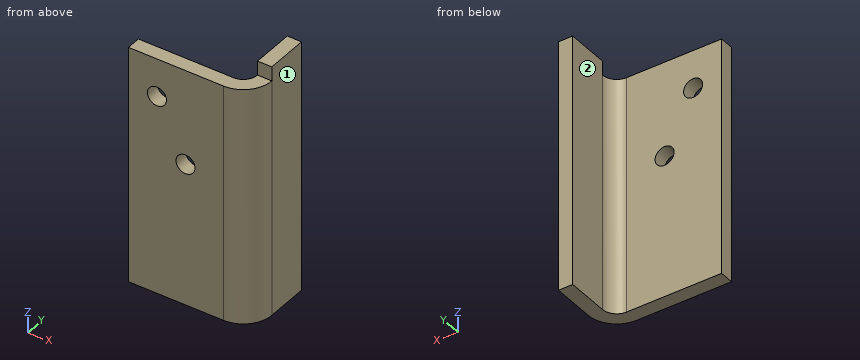
from build123d import *

# Parameters (mm, degrees)
SKETCH1_W               = 20
SKETCH1_H               = 50
SKETCH1_R               = 2
BASE_FLANGE1_DEPTH      = 3
EDGE_FLANGE1_DEPTH      = 50
EDGE_FLANGE1_START      = 3
EDGE_FLANGE1_PROFILE_W  = 53
EDGE_FLANGE1_PROFILE_H  = 9
EDGE_FLANGE1_FLAT_DEPTH = 3


# Sheet-metal steps are written as plain solids
with BuildPart() as part:
    # Sketch1 → Base-Flange1 (new body)
    with BuildSketch(Plane(origin=(0, 0, 0), x_dir=(1, 0, 0), z_dir=(0, 1, 0))):
        Rectangle(SKETCH1_W, SKETCH1_H)
        with Locations(Location((-4, 17, 0), (0, 0, 270))):
            Circle(SKETCH1_R, mode=Mode.SUBTRACT)
        with Locations(Location((2, 5, 0), (0, 0, 270))):
            Circle(SKETCH1_R, mode=Mode.SUBTRACT)
    extrude(amount=-BASE_FLANGE1_DEPTH)

    # Edge-Flange1 bend section (across the edge) → Edge-Flange1 (add)
    with BuildSketch(Plane(origin=(13, 0, 25), x_dir=(-1, 0, 0), z_dir=(0, 0, -1))):
        with BuildLine():
            Line((-3, 3), (0, 3))
            ThreePointArc((0, 3), (0.878679656, 0.878679656), (3, 0))
            Line((3, 0), (3, -3))
            ThreePointArc((3, -3), (-1.242640687, -1.242640687), (-3, 3))
        make_face()
    extrude(amount=EDGE_FLANGE1_DEPTH)

    # Edge-Flange1 profile (on flange) → Edge-Flange1 flat (add)
    with BuildSketch(Plane(origin=(13, 0, 0), x_dir=(0, 0, -1), z_dir=(1, 0, 0)).offset(EDGE_FLANGE1_START)):
        with Locations((1.5, 7.5)):
            Rectangle(EDGE_FLANGE1_PROFILE_W, EDGE_FLANGE1_PROFILE_H)
    extrude(amount=-EDGE_FLANGE1_FLAT_DEPTH)


with BuildPart() as body_2:
    # Mirror1: mirrored copy
    add(part.part.mirror(Plane(origin=(14.5, 7.5, -28), x_dir=(1, 0, 0), z_dir=(0, 0, -1))))


solid = body_2.part
The model under review builds one solid part; all positions refer to its coordinate system, in mm. Face numbers are marked on the shaded views. A direction names the side the tool comes from. Round coordinates to 2 decimals unless told otherwise and drop trailing zeros. Write each loop counter-clockwise with the first axis right and the second up, starting at its lowest first coordinate (ties: lowest second). Pieces come first, ordered by that corner, then holes. Notation, with made-up numbers: (40.5, 22.25) -> (89.5, 22.25) arc R29 ccw to (89.5, 52.25) -> close; hole circle Ø10 at (62, -10). An arc over 180 degrees is marked (long way). Answer as a JSON object with one key per item and string values.
1. We need section A-A on z = -39. State the section outline as (x, y) points.
Results found:
{"outline": "(-10, -3) -> (-6, -3) -> (-6, 0) -> (-10, 0) -> close; (-2, -3) -> (10, -3) arc R6 ccw to (16, 3) -> (16, 12) -> (13, 12) -> (13, 3) arc R3 cw to (10, 0) -> (-2, 0) -> close"}
2. We need section D-D on x = 5.75. State the section outline as (y, z) points.
Results found:
{"outline": "(-3, -81) -> (0, -81) -> (0, -31) -> (-3, -31) -> close"}
3. Machinability: for the marked faces 1 and 2, which of the approach directions +Z, -Z, +X, -X, +Y, -Y give a long, thin tool a straight path to every point of the face, cutting with its end or side? Answer none if there is none.
Results found:
{"face 1": "+Z, -Z, +X, +Y, -Y", "face 2": "+Z, -Z, -X, +Y"}
4. We need section B-B on x = 2. State the section outline as (y, z) points, and give its area (3 significant figures).
Results found:
{"outline": "(-3, -81) -> (0, -81) -> (0, -53) -> (-3, -53) -> close; (-3, -49) -> (0, -49) -> (0, -31) -> (-3, -31) -> close", "area": "138 mm^2"}
5. We need section C-C on y = -2. State the section outline as (x, z) points.
Results found:
{"outline": "(-10, -81) -> (13.32, -81) -> (13.32, -31) -> (-10, -31) -> close; hole circle Ø4 at (-4, -39); hole circle Ø4 at (2, -51)"}
6. Clearance check with flat-ended pins moving along their axes: pin 1 (7 mm diameter, centred on y = 5.5, z = -56.5, fed in from -X); pin 2 (1 mm diameter, centred on x = 7.5, z = -68, fed in from +Y); pin 3 (1 mm diameter, centred on y = 7, z = -67, fed in from -X); pin 4 (2.5 mm diameter, centred on x = 2, z = -51, fed in from -Y). State where each tip first meets the part, or that it passes through.
Results found:
{"pin 1": "stops at x = 12.83", "pin 2": "stops at y = 0", "pin 3": "stops at x = 13", "pin 4": "passes through"}
7. To check wall thickness, follow line 1 along X through (y, z) = (-2.2, -39); line 2 along Y through (x, z) = (-8, -61); line 3 along X through (y, z) = (-0.8, -51). State the ranges of each line that lie inside material, in increasing order.
Results found:
{"line 1": "x = -10 to -6, -2 to 12.99", "line 2": "y = -3 to 0", "line 3": "x = -10 to 0, 4 to 14.64"}
